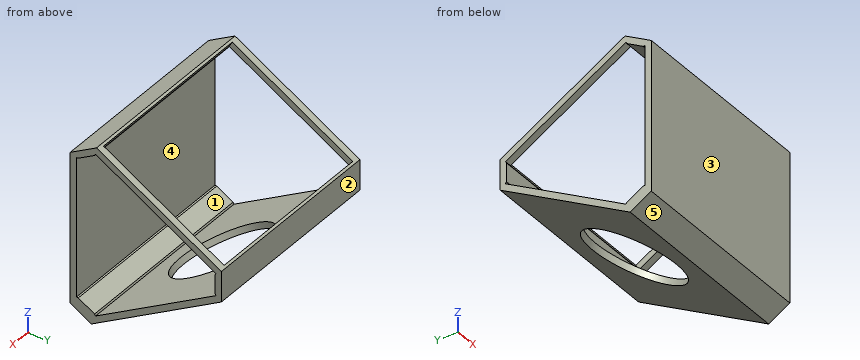
from build123d import *

# Parameters (mm, degrees)
BOSS_EXTRUDE1_DEPTH = 155
SKETCH4_W           = 144
SKETCH4_H           = 111
CUT_EXTRUDE1_DEPTH  = 5
SKETCH5_R           = 38.5
CUT_EXTRUDE2_DEPTH  = 10


with BuildPart() as part:
    # Sketch3 → Boss-Extrude1 (new body)
    with BuildSketch(Plane(origin=(0, 0, 0), x_dir=(0, 0, -1), z_dir=(1, 0, 0))):
        Polygon((58.381197846, 114.119200877), (0.860471904, 14.490381057), (12.979274058, -6.5), (132.75, -6.5), (142.504165125, 10.394709581), (82.618802154, 114.119200877), align=None)
        Polygon((7.5, 12.990381057), (15, 0), (15, -1.5), (126, -1.5), (126, 0), (133.5, 12.990381057), (134.799038106, 13.740381057), (79.299038106, 109.869200877), (78, 109.119200877), (63, 109.119200877), (61.700961894, 109.869200877), (6.200961894, 13.740381057), align=None, mode=Mode.SUBTRACT)
    extrude(amount=BOSS_EXTRUDE1_DEPTH)

    # Sketch4 → Cut-Extrude1 (cut)
    with BuildSketch(Plane(origin=(0, 3.25, 5.629165125), x_dir=(1, 0, 0), z_dir=(0, 0.4999999999999995, 0.8660254037844389))):
        with Locations((77.5, 70.5)):
            Rectangle(SKETCH4_W, SKETCH4_H)
    extrude(amount=-CUT_EXTRUDE1_DEPTH, mode=Mode.SUBTRACT)

    # Sketch5 → Cut-Extrude2 (cut)
    with BuildSketch(Plane(origin=(0, 64.304790967, -111.379165125), x_dir=(-1, 0, 0), z_dir=(0, 0.5000000000000006, -0.8660254037844385))):
        with Locations(Location((-77.5, -2.364637029, 0), (0, 0, 90))):
            Circle(SKETCH5_R)
    extrude(amount=-CUT_EXTRUDE2_DEPTH, mode=Mode.SUBTRACT)


solid = part.part
Geometry: final body of the model. Coordinates: model frame, mm. Face numbers are marked on the shaded views. A direction names the side the tool comes from. Coordinates: 2 decimals unless noted, no trailing zeros. Loops run counter-clockwise (first coordinate to the right, second up) from the corner with the lowest first, then second, coordinate; pieces in that order, holes last. Notation, with made-up numbers: M 78,80 L 115,80 A20 cw 115,108 Z; hole C -32.5,33 d6. An arc over 180 degrees is marked long. One line per item, written item: value. Start each with the question number.
1) Draft query along Z for the marked faces 3, 4 and 5. Return one class per face: released by +Z, released by -Z, zero draft, split by the parting line, or undercut.
2) Reachability of the marked faces 1 and 2 from +Z, -Z, +X, -X, +Y, -Y: full face, straight path, thin tool, end or side. Return the list, or none.
3) Cut plane D-D (z = -48). Return loops of the section in (x, y).
4) Pin query (flat end, axial travel): P1, Ø5, axis at x = 27, y = 36, coming from the -Z side; P2, Ø10, axis at x = 74.5, y = 35.5, coming from the -Z side (1 decimal); P3, Ø2, axis at x = 122, y = 48.5, coming from the -Z side; P4, Ø4, axis at x = 41, y = 99, coming from the +Z side. Return the tip coordinate at first contact, or that it passes through.
5) Cut plane A-A (x = 84.5). Return loops of the section in (y, z), then the cut area to 3 significant figures.
6) Cut plane B-B (x = 141.5). Return loops of the section in (y, z), then the cut area to 3 significant figures.
7) Material intervals for L1, parallel to Y at x = 110, z = -69; L2, parallel to X at y = 87.5, z = -46; L3, parallel to Y at x = 95.5, z = -115, sorted ascending. Write a range as from..to.
8) Cut plane C-C (y = 4). Return loops of the section in (x, z).
Evaluation:
1. face 3: zero draft
1. face 4: undercut
1. face 5: released by -Z
2. face 1: +X, -X
2. face 2: +Z, -Z, +X, -X, +Y
3. outline: M 0,-6.5 L 155,-6.5 L 155,-1.5 L 0,-1.5 Z; M 0,86.14 L 5.5,86.14 L 5.5,96.14 L 0,96.14 Z; M 149.5,86.14 L 155,86.14 L 155,96.14 L 149.5,96.14 Z
4. P1: z = -129.16
4. P2: through
4. P3: z = -121.08
4. P4: z = -84.42
5. outline: M -6.5,-132.75 L 10.39,-142.5 L 29.47,-131.49 L 26.97,-127.16 L 13.74,-134.8 L 12.99,-133.5 L 0,-126 L -1.5,-126 L -1.5,-15 L 0,-15 L 12.99,-7.5 L 16.24,-1.87 L 14.49,-0.86 L -6.5,-12.98 Z; M 92.54,-89.3 L 95.04,-93.63 L 114.12,-82.62 L 114.12,-58.38 L 112.37,-57.37 L 109.12,-63 L 109.12,-78 L 109.87,-79.3 Z
5. area: 1,150 mm^2
6. outline: M -6.5,-132.75 L 10.39,-142.5 L 114.12,-82.62 L 114.12,-58.38 L 112.37,-57.37 L 109.12,-63 L 109.12,-78 L 109.87,-79.3 L 13.74,-134.8 L 12.99,-133.5 L 0,-126 L -1.5,-126 L -1.5,-15 L 0,-15 L 12.99,-7.5 L 16.24,-1.87 L 14.49,-0.86 L -6.5,-12.98 Z
6. area: 1,530 mm^2
7. L1: -6.5..-1.5, 109.12..114.12
7. L2: 0..5.5, 149.5..155
7. L3: -6.5..-1.5
8. outline: M 0,-138.81 L 155,-138.81 L 155,-128.31 L 0,-128.31 Z; M 0,-12.69 L 155,-12.69 L 155,-6.92 L 0,-6.92 Z
